from build123d import *

# Parameters (mm, degrees)
F2_DEPTH = 6.35
F3_D     = 25.4
F4_D     = 88.9


# Not quite as in the source:
# - a length typed as a fraction of an inch, garbled in the dataset ("3 / 203.2 mm" for 3/8 in), is restored


with BuildPart() as f2:
    # F1 (on Front) → F2 (new body)
    with BuildSketch(Plane.XZ):
        with BuildLine():
            ThreePointArc((-47.2755417472, 42.3942574403), (-59.5317634989, 34.5003362533), (-73.8557984397, 31.7890660068))
            ThreePointArc((-73.8557984397, 31.7890660068), (-74.9040664455, 31.8092594153), (-75.9513814682, 31.8582984692))
            ThreePointArc((-75.9513814682, 31.8582984692), (-107.7013814682, 0.1082984692), (-75.9513814682, -31.6417015308))
            ThreePointArc((-75.9513814682, -31.6417015308), (-74.9868907208, -31.6001278987), (-74.0216562697, -31.5830041335))
            ThreePointArc((-74.0216562697, -31.5830041335), (-59.7325831056, -34.2859814401), (-47.4971337693, -42.1458464357))
            ThreePointArc((-47.4971337693, -42.1458464357), (-46.1209982776, -43.530970971), (-44.8176302016, -44.9847765041))
            ThreePointArc((-44.8176302016, -44.9847765041), (0, -63.5000010449), (44.8176302016, -44.9847765041))
            ThreePointArc((44.8176302016, -44.9847765041), (46.2263803756, -43.3976521369), (47.7215078569, -41.8916193935))
            ThreePointArc((47.7215078569, -41.8916193935), (60.0584421445, -34.0280617532), (74.4515791566, -31.4064032457))
            ThreePointArc((74.4515791566, -31.4064032457), (75.1167119815, -31.4211899869), (75.7814841371, -31.4476154228))
            ThreePointArc((75.7814841371, -31.4476154228), (107.7999571445, 2.0780448238), (72.2347193484, 31.814661464))
            ThreePointArc((72.2347193484, 31.814661464), (58.7820372427, 34.8087566031), (47.2755417472, 42.3942574403))
            ThreePointArc((47.2755417472, 42.3942574403), (46.0162162459, 43.6606882414), (44.8176431113, 44.9847615526))
            ThreePointArc((44.8176431113, 44.9847615526), (0, 63.4999989551), (-44.8176431113, 44.9847615526))
            ThreePointArc((-44.8176431113, 44.9847615526), (-46.0162162459, 43.6606882414), (-47.2755417472, 42.3942574403))
        make_face()
    extrude(amount=F2_DEPTH)

    # F3 (through all)
    with Locations(Plane(origin=(0, 0, 0), x_dir=(1, 0, 0), z_dir=(0, 1, 0))):
        with Locations((-76.2, 0), (76.2, 0)):
            Hole(F3_D / 2)

    # F4 (through all)
    with Locations(Plane(origin=(0, 0, 0), x_dir=(1, 0, 0), z_dir=(0, 1, 0))):
        with Locations((0, 0)):
            Hole(F4_D / 2)


solid = f2.part
CAD build for the part. Positions are in the model's coordinates, mm. Coordinates: 2 decimals unless noted, no trailing zeros. Write each loop counter-clockwise with the first axis right and the second up, starting at its lowest first coordinate (ties: lowest second). Pieces come first, ordered by that corner, then holes. Notation, with made-up numbers: (23.25, 58.5) - (76.25, 58.5) arc R31 ccw to (76.25, 85.5) - close; hole circle Ø10 at (28.25, -17). An arc over 180 degrees is marked (long way). Use a Markdown table: item, result. Add a question column.
Item 1: Drill centre lines: L1, parallel to Z at x = 0, y = -1.75; L2, parallel to Z at x = -76.2, y = -1.5; L3, parallel to Z at x = 98, y = -4.5. Where is each one in solid material? Low to high. Write a range as from..to.
Item 2: Mould opens along Z. For faces 1 (the face through (-42.397, -3.219, -13.352)), 2 (the face through (46, -6.35, 1)), 3 (the face through (64.086, -3.219, -3.815)), 4 (the face through (0.697, -3.131, 63.496)) say: pulls with the +Z half, pulls with the -Z half, needs draft (parallel to the pull), parting line crosses it, or undercut.
Item 3: Band-saw the part on C-C, the plane z = 7. Give the cut face in (x, y), and give its area (3 significant figures).
Item 4: Band-saw the part on D-D, the plane z = 20.5. Give the cut face in (x, y).
Item 5: Band-saw the part on A-A, the plane y = -2. Give the cut face in (x, z), and give its area (3 significant figures).
Item 6: Band-saw the part on B-B, the plane x = 0. Give the cut face in (y, z), and give its area (3 significant figures).
Item 7: Flat gauge pin, fed straight in: pin 1 (1.5 mm diameter, centred on y = -2.5, z = 17.5, fed in from +X). Where does the tip first touch, or does it go through?
Numbers:
| question | item | result |
|---|---|---|
| 1 | L1 | -63.5..-44.45, 44.45..63.5 |
| 1 | L2 | -31.64..-12.7, 12.7..31.86 |
| 1 | L3 | -22.69..23.29 |
| 2 | face 1 | undercut |
| 2 | face 2 | needs draft |
| 2 | face 3 | undercut |
| 2 | face 4 | pulls with the +Z half |
| 3 | outline | (-106.94, -6.35) - (-86.8, -6.35) - (-86.8, 0) - (-106.94, 0) - close; (-65.6, -6.35) - (-43.9, -6.35) - (-43.9, 0) - (-65.6, 0) - close; (43.9, -6.35) - (65.6, -6.35) - (65.6, 0) - (43.9, 0) - close; (86.8, -6.35) - (107.13, -6.35) - (107.13, 0) - (86.8, 0) - close |
| 3 | area | 533 mm2 |
| 4 | outline | (-100.29, -6.35) - (-39.44, -6.35) - (-39.44, 0) - (-100.29, 0) - close; (39.44, -6.35) - (100.6, -6.35) - (100.6, 0) - (39.44, 0) - close |
| 5 | outline | (-75.95, -31.64) arc R38.1 cw to (-44.82, -44.98) arc R63.5 ccw to (44.82, -44.98) arc R38.01 cw to (75.78, -31.45) arc R31.75 ccw (long way) to (72.23, 31.81) arc R38.09 cw to (44.82, 44.98) arc R63.5 ccw to (-44.82, 44.98) arc R38.09 cw to (-75.95, 31.86) arc R31.75 ccw to start; hole circle Ø25.4 at (-76.2, 0); hole circle Ø88.9 at (0, 0); hole circle Ø25.4 at (76.2, 0) |
| 5 | area | 10,700 mm2 |
| 6 | outline | (-6.35, -63.5) - (0, -63.5) - (0, -44.45) - (-6.35, -44.45) - close; (-6.35, 44.45) - (0, 44.45) - (0, 63.5) - (-6.35, 63.5) - close |
| 6 | area | 242 mm2 |
| 7 | pin 1 | x = 103.26 |
